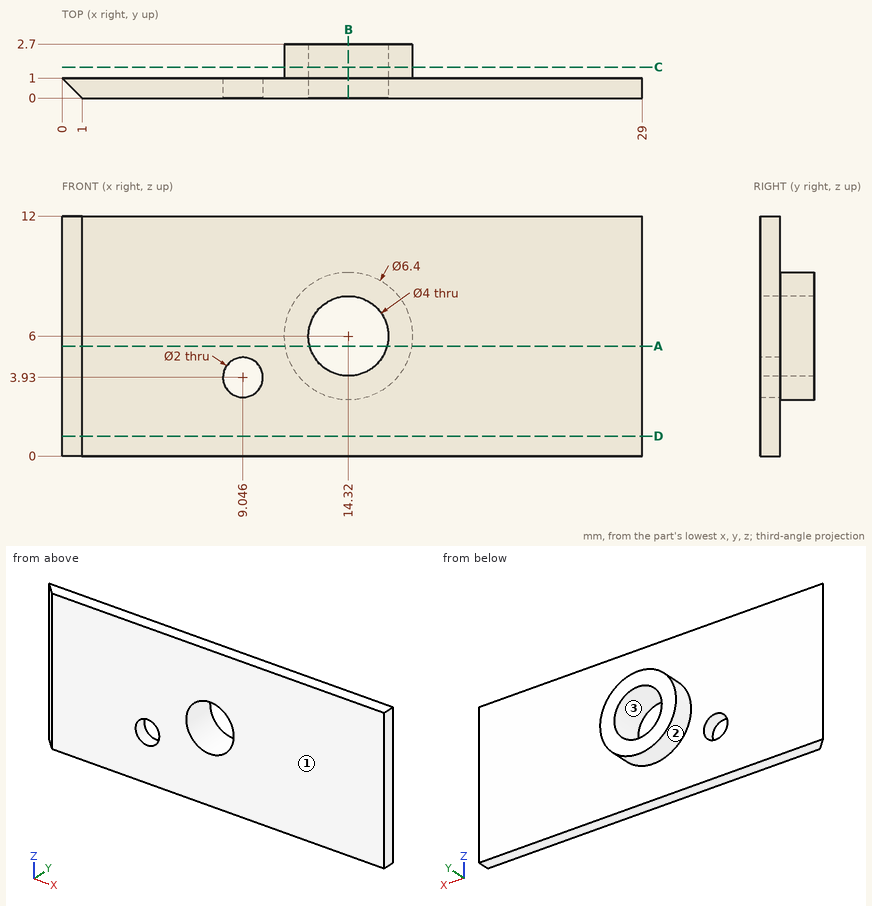
Job drawing, mm, ordinate dimensions from the low corner. One solid piece. Give positions to 0.01 mm unless a question says otherwise; leave off trailing zeros. Loops run counter-clockwise (first coordinate to the right, second up) from the corner with the lowest first, then second, coordinate; pieces in that order, holes last. Notation, with made-up numbers: M 89,38 L 136,38 A12 ccw 136,52 Z; hole C -4.75,50.5 d6. An arc over 180 degrees is marked long. Put each result on its own line as item: value. Start each with the question number.
1) Saw through at A-A (z = 5.5). List the corners of the cut face in (x, y).
2) Probe probe 1 along X at (y, z) = (1.35, 6); probe 2 along Y at (x, z) = (27, 1.5); probe 3 along Z at (x, y) = (12.5, 2.55) (1 decimal). List the from-to ranges inside material, lowest first.
3) Saw through at C-C (y = 1.55). List the corners of the cut face in (x, z), then the cut area to 3 significant figures.
4) Saw through at B-B (x = 14.32). List the corners of the cut face in (y, z), then the cut area to 3 significant figures.
5) Saw through at D-D (z = 1). List the corners of the cut face in (x, y), then the cut area to 3 significant figures.
6) Pull direction Z, two halves, no side cores. Call the marked faces 1, 2 and 3: +Z half, -Z half, draft (parallel to the pull), parting line (faces both ways), or undercut.
7) Flat gauge pins, fed straight in: pin 1 (2.5 mm diameter, centred on x = 9.05, z = 3.93, fed in from +Y); pin 2 (1.5 mm diameter, centred on y = 0.5, z = 8, fed in from -X); pin 3 (5 mm diameter, centred on x = 14.32, z = 6, fed in from -Y). Where does each tip first touch, or does it go through?
Numbers:
1. outline: M 0,1 L 1,0 L 12.38,0 L 12.38,2.7 L 11.16,2.7 L 11.16,1 Z; M 16.26,0 L 29,0 L 29,1 L 17.48,1 L 17.48,2.7 L 16.26,2.7 Z
2. probe 1: 11.12 to 12.32, 16.32 to 17.52
2. probe 2: 0 to 1
2. probe 3: 3.4 to 5.2, 6.8 to 8.6
3. outline: C 14.32,6 d6.4; hole C 14.32,6 d4
3. area: 19.6 mm^2
4. outline: M 0,0 L 1,0 L 1,2.8 L 2.7,2.8 L 2.7,4 L 0,4 Z; M 0,8 L 2.7,8 L 2.7,9.2 L 1,9.2 L 1,12 L 0,12 Z
4. area: 12.1 mm^2
5. outline: M 0,1 L 1,0 L 29,0 L 29,1 Z
5. area: 28.5 mm^2
6. face 1: draft
6. face 2: parting line
6. face 3: undercut
7. pin 1: y = 1
7. pin 2: x = 0
7. pin 3: y = 0
